from build123d import *

# Parameters (mm, degrees)
BOSS_EXTRUDE1_DEPTH = 50.8
FILLET1_R           = 0.762
SKETCH2_R           = 19.05
CUT_EXTRUDE1_DEPTH  = 44.45
SKETCH3_R           = 12.7
CUT_EXTRUDE2_DEPTH  = 66.04


with BuildPart() as part:
    # Sketch1 → Boss-Extrude1 (new body)
    with BuildSketch(Plane.XY):
        Polygon((-21.799999961, -13.97), (-21.799999961, 13.97), (-21.799999961, 64.77), (21.799999961, 64.77), (21.799999961, 13.97), (21.799999961, -13.97), (21.799999961, -77.619999954), (-21.799999961, -77.619999954), align=None)
        Polygon((-15.449999961, 7.62), (-2.54, 7.62), (-2.54, 4.572), (-6.6548, 4.572), (-2.933726616, 0.762), (2.933726616, 0.762), (6.6548, 4.572), (2.54, 4.572), (2.54, 7.62), (15.449999961, 7.62), (15.449999961, -7.62), (-15.449999961, -7.62), align=None, mode=Mode.SUBTRACT)
        Polygon((-13.601813914, -20.32), (0, -40.176776526), (13.601813914, -20.32), align=None, mode=Mode.SUBTRACT)
        Polygon((15.449999961, -28.858349607), (3.848460993, -45.794999977), (15.449999961, -62.731650347), align=None, mode=Mode.SUBTRACT)
        Polygon((-3.848460993, -45.794999977), (-15.449999961, -62.731650347), (-15.449999961, -28.858349607), align=None, mode=Mode.SUBTRACT)
        Polygon((0, -51.413223428), (-13.601813914, -71.269999954), (13.601813914, -71.269999954), align=None, mode=Mode.SUBTRACT)
    extrude(amount=BOSS_EXTRUDE1_DEPTH)

    # Fillet1
    fillet1_edges = [part.edges().sort_by_distance(p)[0] for p in [
        (2.54, 7.62, 25.4),
        (2.54, 4.572, 25.4),
        (6.6548, 4.572, 25.4),
        (2.933726616, 0.762, 25.4),
        (-2.933726616, 0.762, 25.4),
        (-6.6548, 4.572, 25.4),
        (-2.54, 4.572, 25.4),
        (-2.54, 7.62, 25.4),
    ]]
    fillet(fillet1_edges, radius=FILLET1_R)

    # Sketch2 → Cut-Extrude1 (cut)
    with BuildSketch(Plane(origin=(0, 64.77, 0), x_dir=(1, 0, 0), z_dir=(0, 1, 0))):
        with Locations(Location((0, -25.4, 0), (0, 0, 270))):
            Circle(SKETCH2_R)
    extrude(amount=-CUT_EXTRUDE1_DEPTH, mode=Mode.SUBTRACT)

    # Sketch3 → Cut-Extrude2 (cut)
    with BuildSketch(Plane(origin=(0, 64.77, 0), x_dir=(1, 0, 0), z_dir=(0, 1, 0))):
        with Locations(Location((0, -25.4, 0), (0, 0, 270))):
            Circle(SKETCH3_R)
    extrude(amount=-CUT_EXTRUDE2_DEPTH, mode=Mode.SUBTRACT)


solid = part.part
Verification items for the finished model (mm, model axes). A direction names the side the tool comes from. Round coordinates to 2 decimals unless told otherwise and drop trailing zeros. Order: outer loops, then holes, each group sorted by start corner. A loop starts at its lowest first (then second) coordinate and runs counter-clockwise, first axis right, second up.
1. Section check D-D on y = 13. Record the cut outline in (x, z), then the cut area to 3 significant figures.
Final values:
outline: (-21.8, 0) - (21.8, 0) - (21.8, 50.8) - (-21.8, 50.8) - close; hole circle Ø25.4 at (0, 25.4)
area: 1,710 mm2
2. Section check A-A on z = 25.4. Record the cut outline in (x, y) (3 decimals).
Final values:
outline: (-21.8, -77.62) - (21.8, -77.62) - (21.8, 64.77) - (19.05, 64.77) - (19.05, 20.32) - (12.7, 20.32) - (12.7, 7.62) - (15.45, 7.62) - (15.45, -7.62) - (-15.45, -7.62) - (-15.45, 7.62) - (-12.7, 7.62) - (-12.7, 20.32) - (-19.05, 20.32) - (-19.05, 64.77) - (-21.8, 64.77) - close; hole (-15.45, -62.732) - (-3.848, -45.795) - (-15.45, -28.858) - close; hole (-13.602, -71.27) - (13.602, -71.27) - (0, -51.413) - close; hole (-13.602, -20.32) - (0, -40.177) - (13.602, -20.32) - close; hole (3.848, -45.795) - (15.45, -62.732) - (15.45, -28.858) - close
3. Section check B-B on y = -6. Record the cut outline in (x, z), then the cut area to 3 significant figures.
Final values:
outline: (-21.8, 0) - (-15.45, 0) - (-15.45, 50.8) - (-21.8, 50.8) - close; (15.45, 0) - (21.8, 0) - (21.8, 50.8) - (15.45, 50.8) - close
area: 645 mm2
4. Release check for a two-part mould opening along Y. For faces 4 (the flat face through (9.73, -37.21, 25.04)), 5 (the flat face through (0, 10, 0)) record: +Y half, -Y half, draft (parallel to the pull), parting line (faces both ways), or undercut.
Final values:
face 4: undercut
face 5: draft
5. Access from +Z, -Z, +X, -X, +Y, -Y to the whole of each face (thin tool, end or side, straight path). Record for faces 1 (the flat face through (-15.45, 0, 25)), 2 (the cylindrical face through (12.592, 12.851, 23.747)), 3 (the flat face through (-21.8, -5, 25)).
Final values:
face 1: +Z, -Z
face 2: +Y
face 3: +Z, -Z, -X, +Y, -Y
6. Thickness scan on L1, parallel to Y at x = -6, z = 40; L2, parallel to X at y = 54, z = 25.4; L3, parallel to X at y = -42, z = 40.5. Record the ranges inside material, lowest first.
Final values:
L1: y = -77.62 to -71.27, -60.17 to -48.94, -42.65 to -31.42, -20.32 to -7.62, 7.62 to 20.32
L2: x = -21.8 to -19.05, 19.05 to 21.8
L3: x = -21.8 to -15.45, -6.45 to 6.45, 15.45 to 21.8
7. Section check C-C on x = -10.5. Record the cut outline in (y, z), then the cut area to 3 significant figures.
Final values:
outline: (-77.62, 0) - (-71.27, 0) - (-71.27, 50.8) - (-77.62, 50.8) - close; (-66.74, 0) - (-55.51, 0) - (-55.51, 50.8) - (-66.74, 50.8) - close; (-36.08, 0) - (-24.85, 0) - (-24.85, 50.8) - (-36.08, 50.8) - close; (-20.32, 0) - (-7.62, 0) - (-7.62, 50.8) - (-20.32, 50.8) - close; (7.62, 0) - (64.77, 0) - (64.77, 9.5) - (20.32, 9.5) - (20.32, 18.26) - (7.62, 18.26) - close; (7.62, 32.54) - (20.32, 32.54) - (20.32, 41.3) - (64.77, 41.3) - (64.77, 50.8) - (7.62, 50.8) - close
area: 3,420 mm2
8. Go/stop test with flat-tipped pins: P1, Ø1.2, axis at x = 4, z = 40.5, coming from the +Y side; P2, Ø23, axis at x = 0, z = 25.4, coming from the +Y side. Record where each tip stops, or that it passes through.
Final values:
P1: stops at y = 20.32
P2: stops at y = -7.62
